Autodesk Inventor part; units mm, degrees
ref_plane "YZ Plane" through (0, 0, 0) normal (1, 0, 0) x (0, 1, 0)
ref_plane "XZ Plane" through (0, 0, 0) normal (0, 1, 0) x (-1, 0, 0)
ref_plane "XY Plane" through (0, 0, 0) normal (0, 0, 1) x (1, 0, 0)
sketch "Sketch1" plane through (0, 0, 0) normal (0, 1, 0) x (-1, 0, 0)
  circle A0 centre (0, 0) radius 24
  dimension "d0" = 48
extrude "Extrusion1" add sketch "Sketch1" along normal blind 3.96
sketch "Sketch2" plane through (0, 3.96, 0) normal (0, 1, 0) x (1, 0, 0)
  circle A0 centre (0, 0) radius 29
  dimension "d3" = 58
extrude "Extrusion2" add sketch "Sketch2" along normal blind 7
sketch "Sketch3" plane through (0, 10.96, 0) normal (0, 1, 0) x (1, 0, 0)
  circle A0 centre (0, 0) radius 24
  dimension "d6" = 48
extrude "Extrusion3" add sketch "Sketch3" along normal blind 22
sketch "Sketch4" plane through (0, 32.96, 0) normal (0, 1, 0) x (1, 0, 0)
  circle A0 centre (0, 0) radius 21.5
  dimension "d9" = 43
extrude "Extrusion5" add sketch "Sketch4" along normal blind 2
chamfer "Chamfer1" distance 2.97 angle 40 1 edges at (-24, 32.96, 0) measured on face at (23.9222, 25.6267, 1.9312)
chamfer "Chamfer2" distance 2 angle 45 1 edges at (-21.5, 34.96, 0)
sketch "Sketch7" plane through (0, 0, 0) normal (0, -1, 0) x (1, 0, 0)
  circle A0 centre (0, 0) radius 14
  dimension "d22" = 28
extrude "Extrusion6" cut sketch "Sketch7" against normal through all
chamfer "Chamfer3" distance 4 angle 45 1 edges at (-14, 34.96, 0)
properties part number "00.32.005 \"Bushing\"" material "Steel"
Here's how the part is built. I have some questions about the finished solid (model axes, mm). A direction names the side the tool comes from. Give positions to 0.01 mm unless a question says otherwise; leave off trailing zeros. Write each loop counter-clockwise with the first axis right and the second up, starting at its lowest first coordinate (ties: lowest second). Pieces come first, ordered by that corner, then holes. Notation, with made-up numbers: (65, 40.25) -> (110, 40.25) arc R16 cw to (110, 63.25) -> close; hole circle Ø4 at (15, 27). An arc over 180 degrees is marked (long way). Use one line per item in the form item = value. Start each with the question number.
1. Imagine slicing it at C-C on y = 18.5. List the corners of the cut face in (x, z) for me, plus the area to 3 significant figures.
2. Thinking about a two-plate mould opening in Z: for faces 4 (the face through (-23.977, 20.342, 1.055)), 5 (the face through (13.59, 31.21, -4.28)), 6 (the face through (-11, 3.96, -22)), which applies, +Z half, -Z half, draft (parallel to the pull), parting line (faces both ways), or undercut?
3. Will these pins go through, and if not, where does the flat tip stop? pin 1 Ø8 at (x, y) = (-4, 11) entering from +Z; pin 2 Ø2 at (x, y) = (-21.5, 15.5) entering from -Z; pin 3 Ø5 at (x, y) = (16.5, 25) entering from -Z.
4. If I drill on L1, parallel to Z at x = 0, y = 9.5; L2, parallel to Z at x = 0, y = 12; L3, parallel to Y at x = -12.5, z = -22, over which ranges is the centre line in solid material (lowest first)?
5. On a 3-axis mill with a long thin cutter (end or side, diameter ignored), from which of +Z, -Z, +X, -X, +Y, -Y can I reach the whole of each face in a straight line? I mean faces 1 (the face through (23.977, 1.952, -1.055)), 2 (the face through (5.69, 34.96, 17.24)), 3 (the face through (-11, 10.96, -22)). Say none if no direction works.
Entries:
q1.outline = circle Ø48 at (0, 0); hole circle Ø28 at (0, 0)
q1.area = 1,190 mm²
q2.face_4 = parting line
q2.face_5 = undercut
q2.face_6 = draft
q3.pin_1 = 29
q3.pin_2 = -12.48
q3.pin_3 = -19.49
q4.L1 = -29 to -14, 14 to 29
q4.L2 = -24 to -14, 14 to 24
q4.L3 = 3.96 to 10.96
q5.face_1 = -Y
q5.face_2 = +Z, -Z, +X, -X, +Y
q5.face_3 = +Y
